Autodesk Inventor part; units mm, degrees
ref_plane "YZ Plane" through (0, 0, 0) normal (1, 0, 0) x (0, 1, 0)
ref_plane "XZ Plane" through (0, 0, 0) normal (0, 1, 0) x (-1, 0, 0)
ref_plane "XY Plane" through (0, 0, 0) normal (0, 0, 1) x (1, 0, 0)
sketch "Sketch1" plane through (0, 0, 0) normal (0, 1, 0) x (-1, 0, 0)
  line L0 (49, 50) -> (-49, 50)
  line L1 (-49, 50) -> (-49, -50)
  line L2 (-49, -50) -> (49, -50)
  line L3 (49, -50) -> (49, 50)
  line L4 (49, 50) -> (-49, -50) construction
  line L5 (-49, 50) -> (49, -50) construction
  line L6 (52, -53) -> (-52, -53)
  line L7 (-52, -53) -> (-52, 53)
  line L8 (-52, 53) -> (52, 53)
  line L9 (52, 53) -> (52, -53)
  line L10 (46, 47) -> (-46, 47)
  line L11 (-46, 47) -> (-46, -47)
  line L12 (-46, -47) -> (46, -47)
  line L13 (46, -47) -> (46, 47)
  point P0 (0, 0)
  dimension "d0" = 98
  dimension "d1" = 100
  dimension "d2" = 3
  dimension "d3" = 3
extrude "Extrusion1" add sketch "Sketch1" along normal blind 3 contours L3 L2 L1 L0 | L6 L7 L8 L9 | L13 L12 L11 L10
extrude "Extrusion2" add sketch "Sketch1" against normal blind 3 contours L3 L2 L1 L0
sketch "Sketch2" plane through (0, -3, 0) normal (0, -1, 0) x (1, 0, 0)
  line L0 (-49, -50) -> (49, -50)
  circle A0 centre (49, -50) radius 2.5
  circle A1 centre (-49, -50) radius 2.5
  line L1 (49, 50) -> (49, -50)
  circle A2 centre (49, 50) radius 2.5
  line L2 (49, 50) -> (-49, 50)
  circle A3 centre (-49, 50) radius 2.5
  point P0 (0, 0)
  dimension "d8" = 5
  dimension "d9" = 5
  dimension "d10" = 5
  dimension "d12" = 5
extrude "Extrusion3" cut sketch "Sketch2" against normal blind 4.5
fillet "Fillet1" radius 2 8 edges at (-52, 1.5, 53) (0, 3, 53) (-52, 3, 0) (52, 1.5, 53) (52, 3, 0) (52, 1.5, -53) (0, 3, -53) (-52, 1.5, -53)
properties part number "Lid"
Read the model definition and answer for the solid it produces. Units are mm, in the model's axes. A direction names the side the tool comes from. Coordinates: 2 decimals unless noted, no trailing zeros. Order: outer loops, then holes, each group sorted by start corner. A loop starts at its lowest first (then second) coordinate and runs counter-clockwise, first axis right, second up. Notation, with made-up numbers: (78, 15.5) -> (97, 15.5) arc R10 cw to (97, 21.5) -> close; hole circle Ø8 at (18, 41.25). An arc over 180 degrees is marked (long way). Answer as a JSON object with one key per item and string values.
1) Each of these flat-tipped pins is pushed along its axis until it touches: pin 1 (2.5 mm diameter, centred on x = -48, z = 49.5, fed in from -Y); pin 2 (12 mm diameter, centred on x = -30.5, z = -3, fed in from -Y); pin 3 (2.5 mm diameter, centred on x = -16, y = -1.5, fed in from +Z); pin 4 (3.5 mm diameter, centred on y = -1.5, z = -21, fed in from +X). Where does it stop, or does it pass through?
Model answer:
{"pin 1": "stops at y = 1.5", "pin 2": "stops at y = 0", "pin 3": "stops at z = 50", "pin 4": "stops at x = 52"}
2) A cutting plane is placed at A-A, the plane y = -1.45. Determine the outline of the cut face in (x, z).
Model answer:
{"outline": "(-49, -47.5) arc R2.5 cw to (-46.5, -50) -> (46.5, -50) arc R2.5 cw to (49, -47.5) -> (49, 47.5) arc R2.5 cw to (46.5, 50) -> (-46.5, 50) arc R2.5 cw to (-49, 47.5) -> close; hole (-46, -47) -> (46, -47) -> (46, 47) -> (-46, 47) -> close"}
3) A tool of negligible diameter and unlimited length cuts with its end or side. For faces 4 (the face through (1, 3, 1)), 5 (the face through (-1, -1, 50)), 6 (the face through (49, 1.5, -50)), 7 (the face through (-49, -1, -1)), from which of +Z, -Z, +X, -X, +Y, -Y can it reach the whole face along a straight path? Write none if from no direction.
Model answer:
{"face 4": "+Z, -Z, +X, -X, +Y", "face 5": "+Z, +X, -X, -Y", "face 6": "-Y", "face 7": "+Z, -Z, -X, -Y"}
4) Consider line 1 along X through (y, z) = (-0.9, -24); line 2 along Z through (x, y) = (49, 0.55); line 3 along Z through (x, y) = (-35, -1.15). Determine where each line is inside the solid, lowest interval first. Write a range as from..to.
Model answer:
{"line 1": "x = -49..-46, 46..49", "line 2": "z = -53..-52.5, -47.5..47.5, 52.5..53", "line 3": "z = -50..-47, 47..50"}
5) A cutting plane is placed at C-C, the plane z = 14.5. Determine the outline of the cut face in (x, y), plus the area to 3 significant figures.
Model answer:
{"outline": "(-52, 0) -> (-49, 0) -> (-49, -3) -> (-46, -3) -> (-46, 0) -> (46, 0) -> (46, -3) -> (49, -3) -> (49, 0) -> (52, 0) -> (52, 1) arc R2 ccw to (50, 3) -> (-50, 3) arc R2 ccw to (-52, 1) -> close", "area": "328 mm²"}
6) The mould has two halves that part along Z. Classify faces 1 (the face through (1, -1, -50)), 2 (the face through (49, -1, 1)), 3 (the face through (-49, 1.5, -50)): released by +Z, released by -Z, zero draft, split by the parting line, or undercut.
Model answer:
{"face 1": "released by -Z", "face 2": "zero draft", "face 3": "undercut"}
7) A cutting plane is placed at B-B, the plane x = -24.5. Determine the outline of the cut face in (y, z), plus the area to 3 significant figures.
Model answer:
{"outline": "(-3, -50) -> (0, -50) -> (0, -53) -> (1, -53) arc R2 ccw to (3, -51) -> (3, 51) arc R2 ccw to (1, 53) -> (0, 53) -> (0, 50) -> (-3, 50) -> (-3, 47) -> (0, 47) -> (0, -47) -> (-3, -47) -> close", "area": "334 mm²"}
